Check sheet for the modelled part. Datum: model origin and axes. Units: mm. A direction names the side the tool comes from. Round coordinates to 2 decimals unless told otherwise and drop trailing zeros. Order: outer loops, then holes, each group sorted by start corner. A loop starts at its lowest first (then second) coordinate and runs counter-clockwise, first axis right, second up. Notation, with made-up numbers: (39, 47) -> (79, 47) arc R12 ccw to (79, 52) -> close; hole circle Ø4 at (70.5, -8). An arc over 180 degrees is marked (long way). Answer in a Markdown table with one row per item.
from build123d import *

# Parameters (mm, degrees)
DODANIE_WYCI_GNI_CIE1_DEPTH                       = 8
POG_BIENIE_STO_KOWE_POD_M3_WKR_T_DO_2_COUNT       = 2
POG_BIENIE_STO_KOWE_POD_M3_WKR_T_DO_2_PITCH       = 35
SZYK_LINIOWY2_COUNT                               = 2
SZYK_LINIOWY2_PITCH                               = 58
POG_BIENIE_STO_KOWE_POD_M3_WKR_T_DO_3_D           = 3.2
POG_BIENIE_STO_KOWE_POD_M3_WKR_T_DO_3_DEPTH       = 40
POG_BIENIE_STO_KOWE_POD_M3_WKR_T_DO_3_CSINK_D     = 6.3
POG_BIENIE_STO_KOWE_POD_M3_WKR_T_DO_3_CSINK_ANGLE = 90
POG_BIENIE_STO_KOWE_POD_M3_WKR_T_DO_3_TIP         = 0.96137699


with BuildPart() as part:
    # Szkic1 → Dodanie-wyciągnięcie1 (new, symmetric)
    with BuildSketch(Plane.XY):
        Polygon((35, 0), (0, 0), (0, 156), (60, 156), align=None)
    dodanie_wyci_gni_cie1 = extrude(amount=DODANIE_WYCI_GNI_CIE1_DEPTH, both=True)

    # Lustro1: Dodanie-wyciągnięcie1 across plane
    add(dodanie_wyci_gni_cie1.mirror(Plane(origin=(0, 0, 8), x_dir=(0, 0, 1), z_dir=(1, 0, 0))))

    # Szkic5 → Pog_bienie sto_kowe pod M3 wkr_t do cz_c (revolve, cut)
    with BuildSketch(Plane(origin=(29, 101, -8), x_dir=(0, 1, 0), z_dir=(1, 0, 0))):
        Polygon((0, 0), (0, 40.96137699), (1.6, 40), (1.6, 1.55), (3.15, 0), align=None)
    pog_bienie_sto_kowe_pod_m3_wkr_t_do_cz_c = revolve(axis=Axis((29, 101, -14.35), (0, 0, 1)), mode=Mode.SUBTRACT)

    # Pog_bienie sto_kowe pod M3 wkr_t do  2: Pog_bienie sto_kowe pod M3 wkr_t do cz_c ×2
    with Locations(*[(0, i * POG_BIENIE_STO_KOWE_POD_M3_WKR_T_DO_2_PITCH, 0) for i in range(1, POG_BIENIE_STO_KOWE_POD_M3_WKR_T_DO_2_COUNT)]):
        add(pog_bienie_sto_kowe_pod_m3_wkr_t_do_cz_c, mode=Mode.SUBTRACT)

    # Szyk liniowy2: Pog_bienie sto_kowe pod M3 wkr_t do cz_c ×2
    with Locations(*[(-i * SZYK_LINIOWY2_PITCH, 0, 0) for i in range(1, SZYK_LINIOWY2_COUNT)]):
        add(pog_bienie_sto_kowe_pod_m3_wkr_t_do_cz_c, mode=Mode.SUBTRACT)

    # Szyk liniowy2 copy 1 sketch → Szyk liniowy2 copy 1 (revolve, cut)
    with BuildSketch(Plane(origin=(-29, 136, -8), x_dir=(0, 1, 0), z_dir=(1, 0, 0))):
        Polygon((0, 0), (0, 40.96137699), (1.6, 40), (1.6, 1.55), (3.15, 0), align=None)
    revolve(axis=Axis((-29, 136, -14.35), (0, 0, 1)), mode=Mode.SUBTRACT)

    # Pog_bienie sto_kowe pod M3 wkr_t do  3
    with Locations(Plane(origin=(-255, 172, 61), x_dir=(1, 0, 0), z_dir=(0, 1, 0))):
        with Locations((295, 61), (284, 28), (226, 28), (226, 48), (255, 61), (215, 61), (284, 48)):
            CounterSinkHole(POG_BIENIE_STO_KOWE_POD_M3_WKR_T_DO_3_D / 2, POG_BIENIE_STO_KOWE_POD_M3_WKR_T_DO_3_CSINK_D / 2, depth=POG_BIENIE_STO_KOWE_POD_M3_WKR_T_DO_3_DEPTH, counter_sink_angle=POG_BIENIE_STO_KOWE_POD_M3_WKR_T_DO_3_CSINK_ANGLE)
            with Locations((0, 0, -(POG_BIENIE_STO_KOWE_POD_M3_WKR_T_DO_3_DEPTH + POG_BIENIE_STO_KOWE_POD_M3_WKR_T_DO_3_TIP / 2))):  # 118° drill point
                Cone(0, POG_BIENIE_STO_KOWE_POD_M3_WKR_T_DO_3_D / 2, POG_BIENIE_STO_KOWE_POD_M3_WKR_T_DO_3_TIP, mode=Mode.SUBTRACT)


solid = part.part
Item 1: Cross-section at D-D (y = 117). Record the boundary of the cut face in (x, z).
Result sheet:
| item | result |
|---|---|
| outline | (-53.75, -8) -> (53.75, -8) -> (53.75, 8) -> (-53.75, 8) -> close |
Item 2: Set-up check for faces 5 (the cylindrical face through (-38.82, 143.83, -1.08)), 6 (the flat face through (1, 156, 2)): record each of +Z, -Z, +X, -X, +Y, -Y from which the full face is reachable in a straight line by a thin tool's end or side.
Result sheet:
| item | result |
|---|---|
| face 5 | +Y |
| face 6 | +Z, -Z, +X, -X, +Y |
Item 3: Scan lines: line 1 (Y direction, x = 29, z = -5); line 2 (X direction, y = 101, z = 3.75); line 3 (X direction, y = 102, z = 4.75). Record each from-to range of solid material in increasing order. Write a range as [from, to].
Result sheet:
| item | result |
|---|---|
| line 1 | y = [0, 99.4], [102.6, 134.4], [137.6, 156] |
| line 2 | x = [-51.19, -30.6], [-27.4, 27.4], [30.6, 51.19] |
| line 3 | x = [-51.35, -30.25], [-27.75, 27.75], [30.25, 51.35] |
Item 4: Cross-section at C-C (x = 45). Record the boundary of the cut face in (y, z), and give its area (3 significant figures).
Result sheet:
| item | result |
|---|---|
| outline | (62.4, -8) -> (156, -8) -> (156, 8) -> (62.4, 8) -> close |
| area | 1,500 mm^2 |
Item 5: Depth check by flat-ended pin: P1, Ø4, axis at x = 0, z = 0, coming from the +Y side; P2, Ø3, axis at x = 40, z = 0, coming from the +Y side; P3, Ø1.9, axis at x = -40, z = 0, coming from the +Y side; P4, Ø2.5, axis at x = 29, y = 101, coming from the +Z side. Enter the tip coordinate at first touch or a pass-through.
Result sheet:
| item | result |
|---|---|
| P1 | stops at y = 156 |
| P2 | stops at y = 131.94 |
| P3 | stops at y = 131.61 |
| P4 | passes through |
Item 6: Cross-section at B-B (y = 101). Record the boundary of the cut face in (x, z).
Result sheet:
| item | result |
|---|---|
| outline | (-51.19, -8) -> (-32.15, -8) -> (-30.6, -6.45) -> (-30.6, 8) -> (-51.19, 8) -> close; (-27.4, -6.45) -> (-25.85, -8) -> (25.85, -8) -> (27.4, -6.45) -> (27.4, 8) -> (-27.4, 8) -> close; (30.6, -6.45) -> (32.15, -8) -> (51.19, -8) -> (51.19, 8) -> (30.6, 8) -> close |
Item 7: Mould release check, pull along X, two halves, no side actions. Record for faces 1 (the conical face through (-0.278, 131.206, -0.012)), 2 (the cylindrical face through (1.27, 143.83, 0.97)), 3 (the flat face through (47.675, 79.092, 0.112)), 4 (the flat face through (-1, 79, 8)): pulls with the +X half, pulls with the -X half, needs draft (parallel to the pull), parting line crosses it, or undercut.
Result sheet:
| item | result |
|---|---|
| face 1 | undercut |
| face 2 | undercut |
| face 3 | pulls with the +X half |
| face 4 | needs draft |
Item 8: Cross-section at A-A (y = 136). Record the boundary of the cut face in (x, z).
Result sheet:
| item | result |
|---|---|
| outline | (-56.79, -8) -> (-32.15, -8) -> (-30.6, -6.45) -> (-30.6, 8) -> (-56.79, 8) -> close; (-27.4, -6.45) -> (-25.85, -8) -> (25.85, -8) -> (27.4, -6.45) -> (27.4, 8) -> (-27.4, 8) -> close; (30.6, -6.45) -> (32.15, -8) -> (56.79, -8) -> (56.79, 8) -> (30.6, 8) -> close; hole circle Ø3.2 at (-40, 0); hole circle Ø3.2 at (0, 0); hole circle Ø3.2 at (40, 0) |
